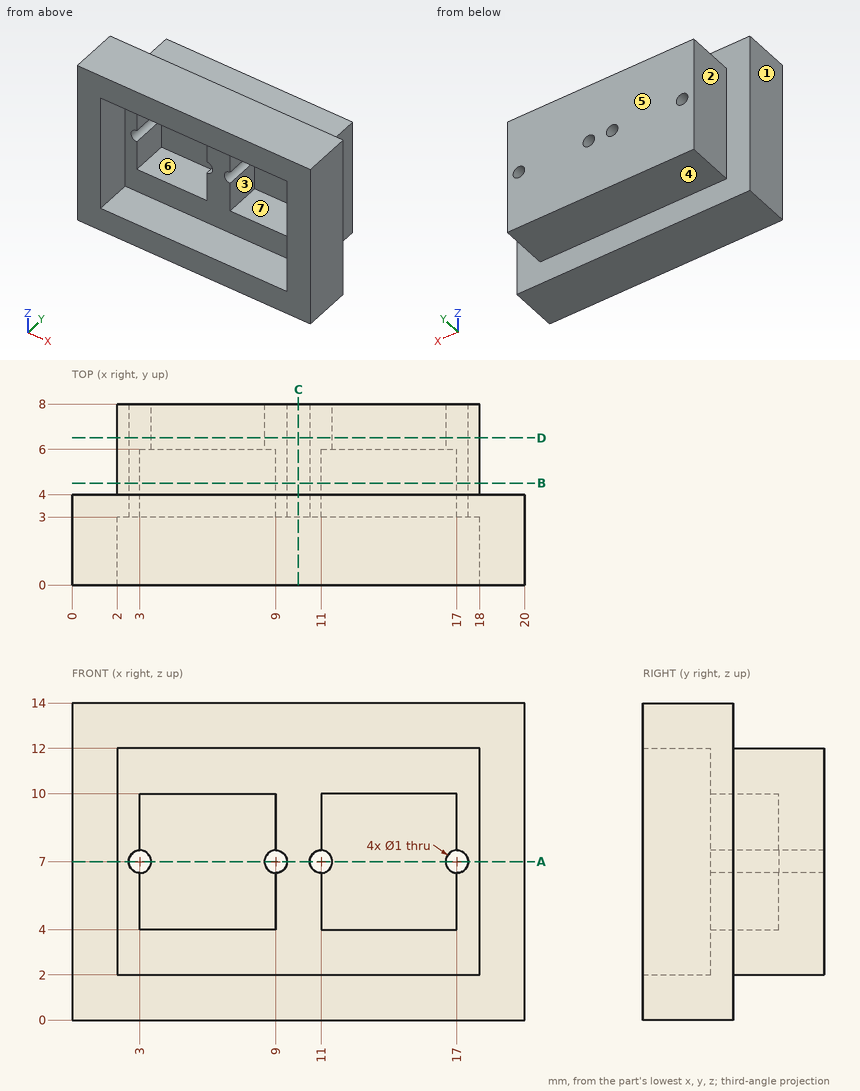
The drawing under review shows one solid part. Ordinate dimensions are in mm from its lowest x, y, z. A direction names the side the tool comes from. Round coordinates to 2 decimals unless told otherwise and drop trailing zeros. Loops run counter-clockwise (first coordinate to the right, second up) from the corner with the lowest first, then second, coordinate; pieces in that order, holes last. Notation, with made-up numbers: (30, 44) - (67, 44) arc R24 cw to (67, 80) - close; hole circle Ø11 at (30, 79). An arc over 180 degrees is marked (long way). Use a Markdown table: item, result. Add a question column.
Q1. Machinability: for the marked faces 1, 2 and 3, which of the approach directions +Z, -Z, +X, -X, +Y, -Y give a long, thin tool a straight path to every point of the face, cutting with its end or side? Answer none if there is none.
Q2. For probe 1 along X at (y, z) = (6.6, 7); probe 2 along X at (y, z) = (2.75, 3.5); probe 3 along Z at (x, y) = (13, 4.5), list the stretches that pass through material, from the lowest coordinate up.
Q3. Add section D-D (y = 6.5). State the section outline as (x, z) points, plus the area to 3 significant figures.
Q4. Insertion check: pin 1 Ø3 at (y, z) = (4, 8.5) entering from -X; pin 2 Ø4.5 at (y, z) = (6.5, 8) entering from -X; pin 3 Ø5 at (x, z) = (15, 8.5) entering from -Y; pin 4 Ø0.8 at (y, z) = (5, 8.5) entering from +X. Each pin has a flat end and moves straight along its axis. Give the tip position at first contact, or say it passes through.
Q5. Add section A-A (z = 7). State the section outline as (x, y) points.
Q6. Add section C-C (x = 10). State the section outline as (y, z) points, plus the area to 3 significant figures.
Q7. Add section B-B (y = 4.5). State the section outline as (x, z) points, plus the area to 3 significant figures.
Q8. The part is to be moulded in two halves that separate along Z. For the marked faces 4, 5, 6 and 7, say which applies: pulls with the +Z half, pulls with the -Z half, needs draft (parallel to the pull), parting line crosses it, or undercut.
Worked answers:
| question | item | result |
|---|---|---|
| 1 | face 1 | +Z, -Z, -X, +Y, -Y |
| 1 | face 2 | +Z, -Z, -X, +Y |
| 1 | face 3 | -Y |
| 2 | probe 1 | 2 to 2.5, 3.5 to 8.5, 9.5 to 10.5, 11.5 to 16.5, 17.5 to 18 |
| 2 | probe 2 | 0 to 2, 18 to 20 |
| 2 | probe 3 | 2 to 4, 10 to 12 |
| 3 | outline | (2, 2) - (18, 2) - (18, 12) - (2, 12) - close; hole circle Ø1 at (3, 7); hole circle Ø1 at (9, 7); hole circle Ø1 at (11, 7); hole circle Ø1 at (17, 7) |
| 3 | area | 157 mm² |
| 4 | pin 1 | x = 0 |
| 4 | pin 2 | x = 2 |
| 4 | pin 3 | y = 3 |
| 4 | pin 4 | x = 18 |
| 5 | outline | (0, 0) - (2, 0) - (2, 3) - (2.5, 3) - (2.5, 8) - (2, 8) - (2, 4) - (0, 4) - close; (3.5, 6) - (8.5, 6) - (8.5, 8) - (3.5, 8) - close; (9.5, 3) - (10.5, 3) - (10.5, 8) - (9.5, 8) - close; (11.5, 6) - (16.5, 6) - (16.5, 8) - (11.5, 8) - close; (17.5, 3) - (18, 3) - (18, 0) - (20, 0) - (20, 4) - (18, 4) - (18, 8) - (17.5, 8) - close |
| 6 | outline | (0, 0) - (4, 0) - (4, 2) - (8, 2) - (8, 12) - (4, 12) - (4, 14) - (0, 14) - (0, 12) - (3, 12) - (3, 2) - (0, 2) - close |
| 6 | area | 66.0 mm² |
| 7 | outline | (2, 2) - (18, 2) - (18, 12) - (2, 12) - close; hole (3, 4) - (9, 4) - (9, 6.5) arc R0.5 ccw to (9, 7.5) - (9, 10) - (3, 10) - (3, 7.5) arc R0.5 ccw to (3, 6.5) - close; hole (11, 4) - (17, 4) - (17, 6.5) arc R0.5 ccw to (17, 7.5) - (17, 10) - (11, 10) - (11, 7.5) arc R0.5 ccw to (11, 6.5) - close |
| 7 | area | 86.4 mm² |
| 8 | face 4 | pulls with the -Z half |
| 8 | face 5 | needs draft |
| 8 | face 6 | undercut |
| 8 | face 7 | undercut |
